Geometry: final body of the model. Coordinates: model frame, mm. Give positions to 0.01 mm unless a question says otherwise; leave off trailing zeros. Write each loop counter-clockwise with the first axis right and the second up, starting at its lowest first coordinate (ties: lowest second). Pieces come first, ordered by that corner, then holes. Notation, with made-up numbers: M 33,52.5 L 41,52.5 A22 cw 41,77.5 Z; hole C 52,85 d6. An arc over 180 degrees is marked long. Use one line per item in the form item = value. Start each with the question number.
Item 1: Contact query for flat-ended pins moving along their axis: P1, Ø3, axis at x = -5.5, y = -10, coming from the -Z side; P2, Ø1.4, axis at x = 25, y = 15, coming from the -Z side. Output: stop coordinate, or through.
Item 2: Section query B-B on x = 25. Return loops of the section in (y, z).
Item 3: Material intervals for line 1 along Y through (x, z) = (25, 3.4); line 2 along Y through (x, z) = (25, 1.7); line 3 along X through (y, z) = (-16.5, 2.3), sorted ascending. Write a range as from..to.
Item 4: Section query A-A on y = 16. Return loops of the section in (x, z).
from build123d import *

# Parameters (mm, degrees)
SKETCH1_W                                      = 60
SKETCH1_H                                      = 40
BOSS_EXTRUDE1_DEPTH                            = 4
FILLET1_R                                      = 1
CBORE_FOR_2_SOCKET_HEAD_CAP_SCREW1_D           = 2.4384
CBORE_FOR_2_SOCKET_HEAD_CAP_SCREW1_DEPTH       = 15
CBORE_FOR_2_SOCKET_HEAD_CAP_SCREW1_CBORE_D     = 4.7625
CBORE_FOR_2_SOCKET_HEAD_CAP_SCREW1_CBORE_DEPTH = 2.1844
CBORE_FOR_2_SOCKET_HEAD_CAP_SCREW1_TIP         = 0.732569267


with BuildPart() as part:
    # Sketch1 → Boss-Extrude1 (new body)
    with BuildSketch(Plane.XY):
        Rectangle(SKETCH1_W, SKETCH1_H)
    extrude(amount=BOSS_EXTRUDE1_DEPTH)

    # Fillet1
    fillet1_edges = [part.edges().sort_by_distance(p)[0] for p in [
        (0, -20, 0),
        (-30, 0, 0),
        (0, 20, 0),
        (30, 0, 0),
    ]]
    fillet(fillet1_edges, radius=FILLET1_R)

    # CBORE for #2 Socket Head Cap Screw1
    with Locations(Plane(origin=(-25, -16, 0), x_dir=(-1, 0, 0), z_dir=(0, 0, -1))):
        with Locations((0, 0), (0, 32), (-50, 32), (-50, 0)):
            CounterBoreHole(CBORE_FOR_2_SOCKET_HEAD_CAP_SCREW1_D / 2, CBORE_FOR_2_SOCKET_HEAD_CAP_SCREW1_CBORE_D / 2, CBORE_FOR_2_SOCKET_HEAD_CAP_SCREW1_CBORE_DEPTH, depth=CBORE_FOR_2_SOCKET_HEAD_CAP_SCREW1_DEPTH)
            with Locations((0, 0, -(CBORE_FOR_2_SOCKET_HEAD_CAP_SCREW1_DEPTH + CBORE_FOR_2_SOCKET_HEAD_CAP_SCREW1_TIP / 2))):  # 118° drill point
                Cone(0, CBORE_FOR_2_SOCKET_HEAD_CAP_SCREW1_D / 2, CBORE_FOR_2_SOCKET_HEAD_CAP_SCREW1_TIP, mode=Mode.SUBTRACT)


solid = part.part
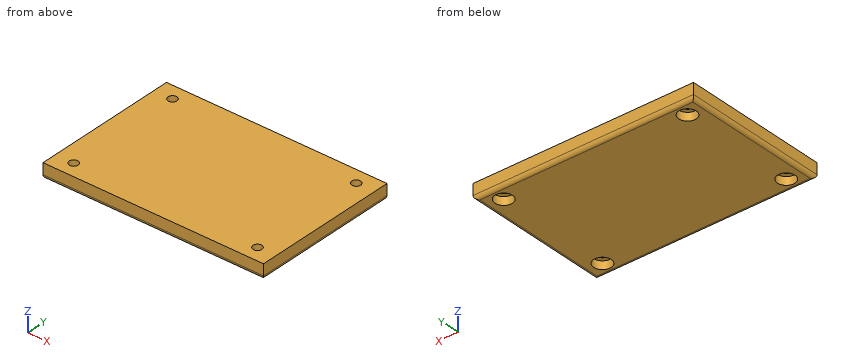
Answer sheet:
q1.P1 = 0
q1.P2 = 2.18
q2.outline = M -20,1 A1 ccw -19,0 L -18.38,0 L -18.38,2.18 L -17.22,2.18 L -17.22,4 L -20,4 Z; M -14.78,2.18 L -13.62,2.18 L -13.62,0 L 13.62,0 L 13.62,2.18 L 14.78,2.18 L 14.78,4 L -14.78,4 Z; M 17.22,2.18 L 18.38,2.18 L 18.38,0 L 19,0 A1 ccw 20,1 L 20,4 L 17.22,4 Z
q3.line_1 = -20..-17.22, -14.78..14.78, 17.22..20
q3.line_2 = -20..-18.38, -13.62..13.62, 18.38..20
q3.line_3 = -30..-26.11, -23.89..23.89, 26.11..30
q4.outline = M -30,1 A1 ccw -29,0 L -27.38,0 L -27.38,2.18 L -26.22,2.18 L -26.22,4 L -30,4 Z; M -23.78,2.18 L -22.62,2.18 L -22.62,0 L 22.62,0 L 22.62,2.18 L 23.78,2.18 L 23.78,4 L -23.78,4 Z; M 26.22,2.18 L 27.38,2.18 L 27.38,0 L 29,0 A1 ccw 30,1 L 30,4 L 26.22,4 Z
